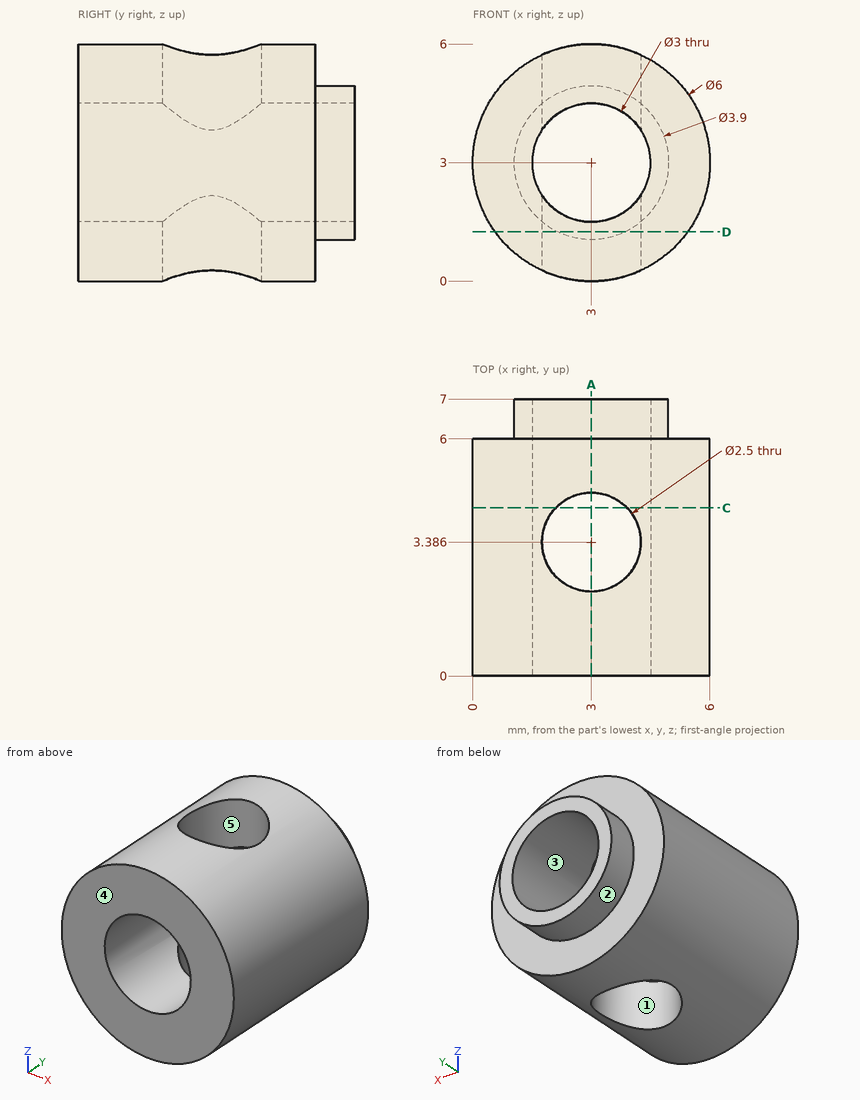
Verification items for this drawing (mm, ordinates from the low corner). A direction names the side the tool comes from. Coordinates: 2 decimals unless noted, no trailing zeros. Loops run counter-clockwise (first coordinate to the right, second up) from the corner with the lowest first, then second, coordinate; pieces in that order, holes last. Notation, with made-up numbers: (54.25, 82) - (63.25, 82) arc R17 ccw to (63.25, 93) - close; hole circle Ø1 at (-13, 27.25). An arc over 180 degrees is marked (long way). Use one line per item in the form item = value. Start each with the question number.
Item 1: Section check D-D, the plane z = 1.25. Enter the section's corners in (x, y).
Item 2: Gauge pin test, flat ends, axial feed: pin 1 (3 mm diameter, centred on x = 5, y = 5.5, fed in from -Z); pin 2 (1 mm diameter, centred on x = 4, y = 5, fed in from +Z); pin 3 (1.5 mm diameter, centred on x = 1.5, y = 4.5, fed in from -Z); pin 4 (2 mm diameter, centred on y = 3, z = 3.5, fed in from +X). Record the tip position at first contact, or that the pin passes through.
Item 3: Section check A-A, the plane x = 3. Enter the section's corners in (y, z), and give its area (3 significant figures).
Item 4: Thickness scan on probe 1 along X at (y, z) = (6.75, 2); probe 2 along Z at (x, y) = (3.25, 2); probe 3 along Y at (x, z) = (0.5, 2). Record the ranges inside material, lowest first.
Item 5: Tool access check on the marked faces 1 and 2. Record the directions out of +Z, -Z, +X, -X, +Y, -Y that give a thin tool (end or side, any length) a straight path to the whole face; none if there is none.
Item 6: Section check C-C, the plane y = 4.25. Enter the section's corners in (x, z).
Item 7: Mould release check, pull along Y, two halves, no side actions. Record for the marked faces 3, 4 and 5: +Y half, -Y half, draft (parallel to the pull), parting line (faces both ways), or undercut.
Computed:
q1.outline = (0.56, 0) - (5.44, 0) - (5.44, 6) - (3.86, 6) - (3.86, 7) - (2.14, 7) - (2.14, 6) - (0.56, 6) - close; hole circle Ø2.5 at (3, 3.39)
q2.pin_1 = 0.04
q2.pin_2 = 5.96
q2.pin_3 = 0.1
q2.pin_4 = 6
q3.outline = (0, 0) - (2.14, 0) - (2.14, 1.5) - (0, 1.5) - close; (0, 4.5) - (2.14, 4.5) - (2.14, 6) - (0, 6) - close; (4.64, 0) - (6, 0) - (6, 1.05) - (7, 1.05) - (7, 1.5) - (4.64, 1.5) - close; (4.64, 4.5) - (7, 4.5) - (7, 4.95) - (6, 4.95) - (6, 6) - (4.64, 6) - close
q3.area = 11.4 mm2
q4.probe_1 = 1.33 to 1.88, 4.12 to 4.67
q4.probe_2 = 0.01 to 1.52, 4.48 to 5.99
q4.probe_3 = 0 to 6
q5.face_1 = +Z, -Z
q5.face_2 = +Y
q6.outline = (2.1, 0.14) - (2.1, 1.8) arc R1.5 cw to (2.1, 4.2) - (2.1, 5.86) arc R3 ccw to start; (3.9, 0.14) arc R3 ccw to (3.9, 5.86) - (3.9, 4.2) arc R1.5 cw to (3.9, 1.8) - close
q7.face_3 = draft
q7.face_4 = -Y half
q7.face_5 = undercut
